Work out the finished part from the listing and answer in its coordinate system (mm). Give positions to 0.01 mm unless a question says otherwise; leave off trailing zeros. Order: outer loops, then holes, each group sorted by start corner. A loop starts at its lowest first (then second) coordinate and runs counter-clockwise, first axis right, second up. Notation, with made-up numbers: M -3.5,14 L 36.5,14 A31 ccw 36.5,48 Z; hole C 38,-5.75 d2. An arc over 180 degrees is marked long. One line per item, written item: value.
from build123d import *

# Parameters (mm, degrees)
BOSS_EXTRUDE3_DEPTH = 3.175


with BuildPart() as part:
    # Sketch1 → Boss-Extrude3 (new body)
    with BuildSketch(Plane(origin=(0, 0, 0), x_dir=(1, 0, 0), z_dir=(0, 1, 0))):
        Polygon((-56.010613502, -81.441915492), (-56.010613502, -84.616915492), (148.179986498, -84.616915492), (148.179986498, -81.441915492), (198.979986498, -81.441915492), (198.979986498, -84.616915492), (249.779986498, -84.616915492), (249.779986498, -81.441915492), (249.779986498, 99.533084508), (249.779986498, 102.708084508), (198.979986498, 102.708084508), (198.979986498, 99.533084508), (148.179986498, 99.533084508), (148.179986498, 102.708084508), (-56.010613502, 102.708084508), (-56.010613502, 99.533084508), (-106.810613502, 99.533084508), (-106.810613502, 102.708084508), (-157.610613502, 102.708084508), (-160.785613502, 102.708084508), (-160.785613502, 99.533084508), (-160.785613502, 74.133084508), (-157.610613502, 74.133084508), (-157.610613502, 48.733084508), (-160.785613502, 48.733084508), (-160.785613502, -30.641915492), (-157.610613502, -30.641915492), (-157.610613502, -56.041915492), (-160.785613502, -56.041915492), (-160.785613502, -81.441915492), (-160.785613502, -84.616915492), (-157.610613502, -84.616915492), (-106.810613502, -84.616915492), (-106.810613502, -81.441915492), align=None)
        Polygon((46.084686498, 15.902033442), (220.245025597, 86.833084508), (-128.0756526, 86.833084508), align=None, mode=Mode.SUBTRACT)
        Polygon((-144.910613502, -61.885466558), (29.249725597, 9.045584508), (-144.910613502, 79.976635573), align=None, mode=Mode.SUBTRACT)
        Polygon((-128.0756526, -68.741915492), (46.084686498, 2.189135573), (220.245025597, -68.741915492), align=None, mode=Mode.SUBTRACT)
        Polygon((62.9196474, 9.045584508), (237.079986498, -61.885466558), (237.079986498, 79.976635573), align=None, mode=Mode.SUBTRACT)
    extrude(amount=BOSS_EXTRUDE3_DEPTH)


solid = part.part
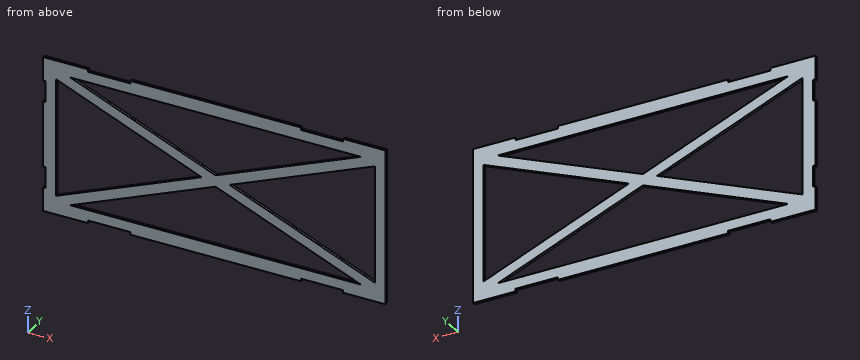
(1) Section C-C, the plane y = 1.6 is taken. Give the number of separate pieces and of enclosed holes in the cut face, then the cut area to 3 significant figures.
Findings:
separate pieces: 1
enclosed holes: 4
area: 26,700 mm^2
(2) Given P1, Ø1, axis at x = -84, y = 1, coming from the -Z side; P2, Ø1.6, axis at y = 2.5, z = 49.5, coming from the -X side, each flat-ended and moving along its own axis, determine where each tip first touches the part or whether it passes through.
Findings:
P1: stops at z = -99.53
P2: stops at x = -157.61
(3) Find the intervals of material crossed by probe 1 along Z at (x, y) = (166, 1.4); probe 2 along Z at (x, y) = (215.5, 2); probe 3 along X at (y, z) = (0.75, -12), in increasing order. Write a range as from..to.
Findings:
probe 1: z = -99.53..-86.83, -64.74..-51.03, 32.94..46.65, 68.74..81.44
probe 2: z = -102.71..-86.83, -84.9..-71.19, 53.1..66.81, 68.74..84.62
probe 3: x = -160.79..-144.91, 22..70.17, 237.08..249.78
(4) Section B-B, the plane x = -36.5 is taken. Give the vertices of the cut face in (y, z) (1 decimal).
Findings:
outline: M 0,-102.7 L 3.2,-102.7 L 3.2,-86.8 L 0,-86.8 Z; M 0,-49.5 L 3.2,-49.5 L 3.2,-35.8 L 0,-35.8 Z; M 0,17.7 L 3.2,17.7 L 3.2,31.4 L 0,31.4 Z; M 0,68.7 L 3.2,68.7 L 3.2,84.6 L 0,84.6 Z
(5) Section A-A, the plane z = -69.5 is taken. Give the vertices of the cut face in (x, y) (3 decimals), then the cut area to 3 significant figures.
Findings:
outline: M -157.611,0 L -144.911,0 L -144.911,3.175 L -157.611,3.175 Z; M -119.187,0 L -85.517,0 L -85.517,3.175 L -119.187,3.175 Z; M 177.686,0 L 211.356,0 L 211.356,3.175 L 177.686,3.175 Z; M 237.08,0 L 249.78,0 L 249.78,3.175 L 237.08,3.175 Z
area: 294 mm^2
